Build history of the part. All positions in model axes, mm. Face numbers are marked on the shaded views. A direction names the side the tool comes from. Round coordinates to 2 decimals unless told otherwise and drop trailing zeros. Write each loop counter-clockwise with the first axis right and the second up, starting at its lowest first coordinate (ties: lowest second). Pieces come first, ordered by that corner, then holes.
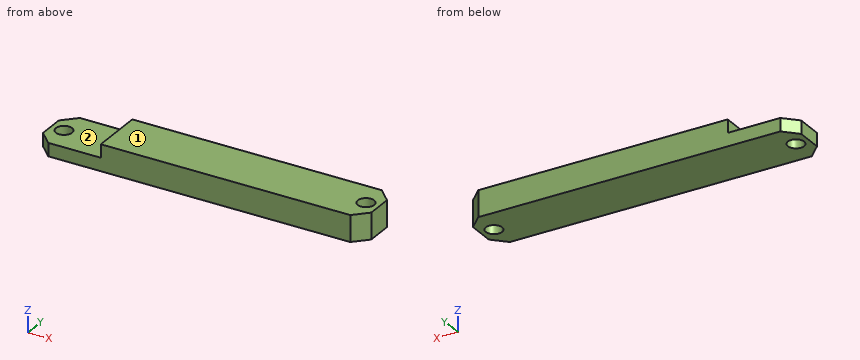
Autodesk Inventor part; units mm, degrees
ref_plane "YZ Plane" through (0, 0, 0) normal (1, 0, 0) x (0, 1, 0)
ref_plane "XZ Plane" through (0, 0, 0) normal (0, 1, 0) x (-1, 0, 0)
ref_plane "XY Plane" through (0, 0, 0) normal (0, 0, 1) x (1, 0, 0)
sketch "スケッチ1" plane through (0, 0, 0) normal (0, 1, 0) x (-1, 0, 0)
  line L0 (-25, -2) -> (25, -2)
  line L1 (25, -2) -> (25, 2)
  line L2 (25, 2) -> (-25, 2)
  line L3 (-25, 2) -> (-25, -2)
  line L4 (-25, -2) -> (25, 2) construction
  line L5 (25, -2) -> (-25, 2) construction
  point P0 (0, 0)
  dimension "d0" = 50
  dimension "d1" = 4
extrude "押し出し1" add sketch "スケッチ1" along normal mid plane 8
sketch "スケッチ2" plane through (0, 0, 0) normal (0, 0, 1) x (1, 0, 0)
  circle A0 centre (-23, 0) radius 1.25
  line L0 (-25, -4) -> (-25, 4)
  circle A1 centre (23, 0) radius 1.25
  line L1 (25, -4) -> (25, 4)
  point P0 (0, 0)
  dimension "d4" = 2.5
  dimension "d5" = 2
  dimension "d14" = 2.5
  dimension "d15" = 2
extrude "押し出し2" cut sketch "スケッチ2" along normal mid plane 5 contours A0
chamfer "面取り1" distance 2 angle 45 1 edges at (-25, 4, 0)
chamfer "面取り2" distance 2 angle 45 1 edges at (-25, -4, 0)
sketch "スケッチ3" plane through (0, 0, 0) normal (0, 0, 1) x (1, 0, 0)
  circle A0 centre (23, 0) radius 1.25
  line L0 (25, -4) -> (25, 4)
  point P0 (0, 0)
  dimension "d16" = 2.5
  dimension "d17" = 2
extrude "押し出し3" cut sketch "スケッチ3" along normal mid plane 5
chamfer "面取り3" distance 2 angle 45 1 edges at (25, 4, 0)
chamfer "面取り4" distance 2 angle 45 1 edges at (25, -4, 0)
sketch "スケッチ4" plane through (0, -4, 0) normal (0, -1, 0) x (1, 0, 0)
  line L0 (-25, -2) -> (-25, 2)
  line L1 (-25, 0) -> (-15, 0)
  line L2 (-15, 0) -> (-15, 2)
  line L3 (-15, 2) -> (-25, 2)
  line L4 (-25, 2) -> (-25, 0)
  point P0 (0, 0)
  dimension "d26" = 10
extrude "押し出し4" cut sketch "スケッチ4" against normal blind 10
properties part number "promo_arm1"
1) Which spindle directions (+Z, -Z, +X, -X, +Y, -Y) get a long thin tool onto all of the face, cutting with end or side? Do the marked faces 1 and 2. Say none if no direction does.
Results:
face 1: +Z, +X, -X, +Y, -Y
face 2: +Z, -X, +Y, -Y
2) Pin check, flat tip, straight feed: pin 1 Ø2.5 at (x, y) = (-18, 1.5) entering from +Z. Stop position of the tip, or through.
Results:
pin 1: stops at z = 0
3) Slice it at A-A (z = 1.2). Write the cut outline in (x, y), plus the area to 3 significant figures.
Results:
outline: (-15, -4) - (23, -4) - (25, -2) - (25, 2) - (23, 4) - (-15, 4) - close; hole circle Ø2.5 at (23, 0)
area: 311 mm2
4) Wall check: L1, parallel to X at y = 0, z = 0.85; L2, parallel to Y at x = 23, z = 0.7; L3, parallel to X at y = 1, z = 1.75. Give the ranges that are in metal, low to high.
Results:
L1: x = -15 to 21.75, 24.25 to 25
L2: y = -4 to -1.25, 1.25 to 4
L3: x = -15 to 22.25, 23.75 to 25
5) Slice it at C-C (z = -0.6). Write the cut outline in (x, y), plus the area to 3 significant figures.
Results:
outline: (-25, -2) - (-23, -4) - (23, -4) - (25, -2) - (25, 2) - (23, 4) - (-23, 4) - (-25, 2) - close; hole circle Ø2.5 at (-23, 0); hole circle Ø2.5 at (23, 0)
area: 382 mm2
6) Slice it at B-B (y = 0). Write the cut outline in (x, z), plus the area to 3 significant figures.
Results:
outline: (-25, -2) - (-24.25, -2) - (-24.25, 0) - (-25, 0) - close; (-21.75, -2) - (21.75, -2) - (21.75, 2) - (-15, 2) - (-15, 0) - (-21.75, 0) - close; (24.25, -2) - (25, -2) - (25, 2) - (24.25, 2) - close
area: 165 mm2
